Here's how the part is built. I have some questions about the finished solid (model axes, mm). A direction names the side the tool comes from. Coordinates: 2 decimals unless noted, no trailing zeros. Loops run counter-clockwise (first coordinate to the right, second up) from the corner with the lowest first, then second, coordinate; pieces in that order, holes last. Notation, with made-up numbers: (-1, 80) -> (8, 80) arc R20 cw to (8, 118) -> close; hole circle Ø3 at (25.25, 58.5). An arc over 180 degrees is marked (long way). Answer as a JSON object with one key per item and string values. Group by question number.
Q1. I want a section at B-B on y = 50. Write out the boundary of the cut face in (x, z).
Q2. I want a section at A-A on z = -7.5. Write out the boundary of the cut face in (x, y), then the cut area to 3 significant figures.
Q3. I need wall thicknesses on line 1 (Y direction, x = 44, z = -9); line 2 (X direction, y = 24.5, z = -4.5); line 3 (Z direction, x = -5, y = 22.5). Which ranges of each line are inside material? Lowest first, please.
Q4. On a 3-axis mill with a long thin cutter (end or side, diameter ignored), from which of +Z, -Z, +X, -X, +Y, -Y can I reach the whole of each face in a straight line? I mean faces 1 (the flat face through (-7.5, 28, -18)), 2 (the cylindrical face through (4.78, 62.4, -24.43)), 3 (the flat face through (1, 13, 0)), 4 (the flat face through (29, 12, -12)), 5 (the cylindrical face through (47.4, -8.77, -36.43)). Say none if no direction works.
Q5. I'm going to push flat-ended pins straight in: pin 1 (8 mm diameter, centred on x = 41.5, z = -32.5, fed in from +Y); pin 2 (16.5 mm diameter, centred on x = 11.5, y = 20.5, fed in from -Z); pin 3 (10 mm diameter, centred on x = 23.5, z = -12, fed in from +Y). Where does each tip first touch, or does it pass through?
Q6. Thinking about a two-plate mould opening in X: for faces 6 (the cylindrical face through (-11, -10, -17)), 7 (the cylindrical face through (6.4, 38.84, 3.43)), 8 (the flat face through (5, 10, 4)), 9 (the flat face through (2.5, 36, -12)), which applies, released by +X, released by -X, zero draft, split by the parting line, or undercut?
Q7. I want a section at D-D on x = -3. Write out the boundary of the cut face in (y, z), then the cut area to 3 significant figures.
Q8. I want a section at C-C on z = -27. Write out the boundary of the cut face in (x, y).
```python
from build123d import *

# Parameters (mm, degrees)
F1_DEPTH    = 4
F3_DEPTH    = 25
F5_DEPTH    = 12
F6_R        = 2
F7_T1_DEPTH = 41
F7_T4_ANGLE = 90
F7_T6_ANGLE = 90


# Not quite as in the source:
# - a fillet or chamfer that OpenCascade refuses, or shapes differently, is made with other operations: its cross-section is extruded or revolved along the edge and cut away or added


with BuildPart() as f1:
    # F0 (on Top) → F1 (new body)
    with BuildSketch(Plane.XY):
        Polygon((7, 12), (7, 63), (-12, 63), (-12, -12), (48, -12), (48, 12), align=None)
    extrude(amount=F1_DEPTH)

    # F2 (on face) → F3 (join)
    with BuildSketch(Plane(origin=(0, 0, 0), x_dir=(1, 0, 0), z_dir=(0, 0, -1))):
        Polygon((48, 12), (-12, 12), (-12, -63), (-7.5, -63), (-7.5, 7.5), (48, 7.5), align=None)
        Polygon((2.5, -63), (7, -63), (7, -12), (48, -12), (48, -7.5), (2.5, -7.5), align=None)
    extrude(amount=F3_DEPTH)

    # F4 (on face) → F5 (join)
    with BuildSketch(Plane(origin=(0, 0, -25), x_dir=(1, 0, 0), z_dir=(0, 0, -1))):
        Polygon((48, 12), (-12, 12), (-12, -63), (-7.5, -63), (-7.5, 7.5), (48, 7.5), align=None)
    extrude(amount=F5_DEPTH)

    # F6
    f6_edges = [f1.edges().sort_by_distance(p)[0] for p in [
        (7, 37.5, 4),
        (-2.5, 63, 4),
        (-12, 25.5, 4),
        (18, -12, 4),
        (48, 0, 4),
        (27.5, 12, 4),
        (-9.75, 63, -37),
        (4.75, 63, -25),
        (48, -9.75, -37),
        (48, 9.75, -25),
        (2.5, 7.5, -12.5),
        (7, 12, -10.5),
        (-12, 63, -16.5),
        (48, -12, -16.5),
        (-12, 25.5, -37),
        (18, -12, -37),
    ]]
    fillet(f6_edges, radius=F6_R)

    # F7: fillet of radius 5 on 1 edges, made by hand

    # F7_s2 → F7_t1 (cut)
    with BuildSketch(Plane.XY.offset(-37)):
        with BuildLine():
            ThreePointArc((-12, -7), (-10.5355339059, -10.5355339059), (-7, -12))
            Line((-7, -12), (-12, -12))
            Line((-12, -12), (-12, -7))
        make_face()
    extrude(amount=F7_T1_DEPTH, mode=Mode.SUBTRACT)

    # F7_s3 → F7_t4 (revolve, cut)
    with BuildSketch(Plane.YZ.offset(-7)):
        with BuildLine():
            ThreePointArc((-10, -37), (-11.4142135624, -36.4142135624), (-12, -35))
            Line((-12, -35), (-12, -37))
            Line((-12, -37), (-10, -37))
        make_face()
    revolve(axis=Axis((-7, -7, -37), (0, 0, -1)), revolution_arc=F7_T4_ANGLE, mode=Mode.SUBTRACT)

    # F7_s5 → F7_t6 (revolve, cut)
    with BuildSketch(Plane.XZ.offset(7)):
        with BuildLine():
            ThreePointArc((-10, 4), (-11.4142135624, 3.4142135624), (-12, 2))
            Line((-12, 2), (-12, 4))
            Line((-12, 4), (-10, 4))
        make_face()
    revolve(axis=Axis((-7, -7, 4), (0, 0, 1)), revolution_arc=F7_T6_ANGLE, mode=Mode.SUBTRACT)


solid = f1.part
```
Result set:
{
 "1": {"outline": "(-12, -35) arc R2 ccw to (-10, -37) -> (-7.5, -37) -> (-7.5, 0) -> (2.5, 0) -> (2.5, -25) -> (7, -25) -> (7, 2) arc R2 ccw to (5, 4) -> (-10, 4) arc R2 ccw to (-12, 2) -> close"},
 "2": {"outline": "(-12, -7) arc R5 ccw to (-7, -12) -> (46, -12) arc R2 ccw to (48, -10) -> (48, -7.5) -> (-7.5, -7.5) -> (-7.5, 63) -> (-10, 63) arc R2 ccw to (-12, 61) -> close; (2.5, 9.5) arc R2 ccw to (4.5, 7.5) -> (48, 7.5) -> (48, 12) -> (9, 12) arc R2 cw to (7, 14) -> (7, 63) -> (2.5, 63) -> close", "area": "1,010 mm²"},
 "3": {"line 1": "y = -12 to -7.5, 7.5 to 12", "line 2": "x = -12 to -7.5, 2.5 to 7", "line 3": "z = 0 to 4"},
 "4": {"face 1": "-Z, +Y", "face 2": "-Z, +X, +Y", "face 3": "-Z", "face 4": "+Z, -Z, +X, +Y", "face 5": "-Z, +X, +Y, -Y"},
 "5": {"pin 1": "stops at y = -7.5", "pin 2": "stops at z = -25", "pin 3": "stops at y = 12"},
 "6": {"face 6": "released by -X", "face 7": "released by +X", "face 8": "zero draft", "face 9": "undercut"},
 "7": {"outline": "(-12, -35) arc R2 ccw to (-10, -37) -> (-7.5, -37) -> (-7.5, 0) -> (63, 0) -> (63, 2) arc R2 ccw to (61, 4) -> (-10, 4) arc R2 ccw to (-12, 2) -> close", "area": "464 mm²"},
 "8": {"outline": "(-12, -7) arc R5 ccw to (-7, -12) -> (46, -12) arc R2 ccw to (48, -10) -> (48, -7.5) -> (-7.5, -7.5) -> (-7.5, 63) -> (-10, 63) arc R2 ccw to (-12, 61) -> close"}
}
